from build123d import *

# Parameters (mm, degrees)
F1_DEPTH = 12.7
F2_R     = 9.525
F3_DEPTH = 34.29
F4_DEPTH = 25.4
F2_R_2   = 25.4
F5_DEPTH = 6.35


with BuildPart() as f1:
    # F0 (on Top) → F1 (new body)
    with BuildSketch(Plane.XY):
        Polygon((-48.986719159, 25.3412460777), (-50.7255351294, 24.7465363945), (-52.3601977854, 21.688304154), (-53.366815822, 18.3699267661), (-52.5578082129, 16.719871907), (-47.6057296253, 11.0468524364), (-43.80914346, 8.4974130761), (-42.2801519731, 7.9744654227), (-37.0147232049, 7.6171909331), (-33.782, 5.0679251692), (-33.782, -5.0679251692), (-37.0147232049, -7.6171909331), (-42.2801519731, -7.9744654227), (-43.80914346, -8.4974130761), (-47.6057296253, -11.0468524364), (-52.5578082129, -16.719871907), (-53.366815822, -18.3699267661), (-52.3601977854, -21.688304154), (-50.7255351294, -24.7465363945), (-48.986719159, -25.3412460777), (-41.4736370284, -25.8510271212), (-36.9863201834, -24.9691669416), (-35.5353802528, -24.2577827562), (-31.559527, -20.7871925925), (-27.4710453735, -20.303918365), (-20.303918365, -27.4710453735), (-20.7871925925, -31.559527), (-24.2577827562, -35.5353802528), (-24.9691669416, -36.9863201834), (-25.8510271212, -41.4736370284), (-25.3412460777, -48.986719159), (-24.7465363945, -50.7255351294), (-21.688304154, -52.3601977854), (-18.3699267661, -53.366815822), (-16.719871907, -52.5578082129), (-11.0468524364, -47.6057296253), (-8.4974130761, -43.80914346), (-7.9744654227, -42.2801519731), (-7.6171909331, -37.0147232049), (-5.0679251692, -33.782), (5.0679251692, -33.782), (7.6171909331, -37.0147232049), (7.9744654227, -42.2801519731), (8.4974130761, -43.80914346), (11.0468524364, -47.6057296253), (16.719871907, -52.5578082129), (18.3699267661, -53.366815822), (21.688304154, -52.3601977854), (24.7465363945, -50.7255351294), (25.3412460777, -48.986719159), (25.8510271212, -41.4736370284), (24.9691669416, -36.9863201834), (24.2577827562, -35.5353802528), (20.7871925925, -31.559527), (20.303918365, -27.4710453735), (27.4710453735, -20.303918365), (31.559527, -20.7871925925), (35.5353802528, -24.2577827562), (36.9863201834, -24.9691669416), (41.4736370284, -25.8510271212), (48.986719159, -25.3412460777), (50.7255351294, -24.7465363945), (52.3601977854, -21.688304154), (53.366815822, -18.3699267661), (52.5578082129, -16.719871907), (47.6057296253, -11.0468524364), (43.80914346, -8.4974130761), (42.2801519731, -7.9744654227), (37.0147232049, -7.6171909331), (33.782, -5.0679251692), (33.782, 5.0679251692), (37.0147232049, 7.6171909331), (42.2801519731, 7.9744654227), (43.80914346, 8.4974130761), (47.6057296253, 11.0468524364), (52.5578082129, 16.719871907), (53.366815822, 18.3699267661), (52.3601977854, 21.688304154), (50.7255351294, 24.7465363945), (48.986719159, 25.3412460777), (41.4736370284, 25.8510271212), (36.9863201834, 24.9691669416), (35.5353802528, 24.2577827562), (31.559527, 20.7871925925), (27.4710453735, 20.303918365), (20.303918365, 27.4710453735), (20.7871925925, 31.559527), (24.2577827562, 35.5353802528), (24.9691669416, 36.9863201834), (25.8510271212, 41.4736370284), (25.3412460777, 48.986719159), (24.7465363945, 50.7255351294), (21.688304154, 52.3601977854), (18.3699267661, 53.366815822), (16.719871907, 52.5578082129), (11.0468524364, 47.6057296253), (8.4974130761, 43.80914346), (7.9744654227, 42.2801519731), (7.6171909331, 37.0147232049), (5.0679251692, 33.782), (-5.0679251692, 33.782), (-7.6171909331, 37.0147232049), (-7.9744654227, 42.2801519731), (-8.4974130761, 43.80914346), (-11.0468524364, 47.6057296253), (-16.719871907, 52.5578082129), (-18.3699267661, 53.366815822), (-21.688304154, 52.3601977854), (-24.7465363945, 50.7255351294), (-25.3412460777, 48.986719159), (-25.8510271212, 41.4736370284), (-24.9691669416, 36.9863201834), (-24.2577827562, 35.5353802528), (-20.7871925925, 31.559527), (-20.303918365, 27.4710453735), (-27.4710453735, 20.303918365), (-31.559527, 20.7871925925), (-35.5353802528, 24.2577827562), (-36.9863201834, 24.9691669416), (-41.4736370284, 25.8510271212), align=None)
        Polygon((-6.457554456, 6.1279886028), (-5.0423575535, 7.3366771559), (-3.4067913067, 8.2247200336), (-1.622328418, 8.7533028893), (0.2330374214, 8.8993240645), (2.0782189459, 8.6564005578), (3.8325695574, 8.0351529003), (5.4194220185, 7.0627288788), (6.7694179402, 5.7816284228), (7.8235568446, 4.247847459), (8.5357689507, 2.5284119549), (8.8749315621, 0.6984712932), (8.8262133252, -1.1619911548), (8.3917463583, -2.9716744665), (7.5905194232, -4.6514766054), (6.457554456, -6.1279886028), (5.0423575535, -7.3366771559), (3.4067913067, -8.2247200336), (1.622328418, -8.7533028893), (-0.2330374214, -8.8993240645), (-2.0782189459, -8.6564005578), (-3.8325695574, -8.0351529003), (-5.4194220185, -7.0627288788), (-6.7694179402, -5.7816284228), (-7.8235568446, -4.247847459), (-8.5357689507, -2.5284119549), (-8.8749315621, -0.6984712932), (-8.8262133252, 1.1619911548), (-8.3917463583, 2.9716744665), (-7.5905194232, 4.6514766054), align=None, mode=Mode.SUBTRACT)
        Polygon((-3.4067913067, 8.2247200336), (-5.0423575535, 7.3366771559), (-6.457554456, 6.1279886028), (-7.5905194232, 4.6514766054), (-8.3917463583, 2.9716744665), (-8.8262133252, 1.1619911548), (-8.8749315621, -0.6984712932), (-8.5357689507, -2.5284119549), (-7.8235568446, -4.247847459), (-6.7694179402, -5.7816284228), (-5.4194220185, -7.0627288788), (-3.8325695574, -8.0351529003), (-2.0782189459, -8.6564005578), (-0.2330374214, -8.8993240645), (1.622328418, -8.7533028893), (3.4067913067, -8.2247200336), (5.0423575535, -7.3366771559), (6.457554456, -6.1279886028), (7.5905194232, -4.6514766054), (8.3917463583, -2.9716744665), (8.8262133252, -1.1619911548), (8.8749315621, 0.6984712932), (8.5357689507, 2.5284119549), (7.8235568446, 4.247847459), (6.7694179402, 5.7816284228), (5.4194220185, 7.0627288788), (3.8325695574, 8.0351529003), (2.0782189459, 8.6564005578), (0.2330374214, 8.8993240645), (-1.622328418, 8.7533028893), align=None)
    extrude(amount=F1_DEPTH)

    # F2 (on face) → F3 (join)
    with BuildSketch(Plane.XY.offset(12.7)):
        Circle(F2_R)
        with BuildLine():
            ThreePointArc((1.7960512242, 2.921), (2.9930503377, 1.6732276223), (3.429, 0))
            ThreePointArc((3.429, 0), (-1.6732276223, -2.9930503377), (-1.7960512242, 2.921))
            ThreePointArc((-1.7960512242, 2.921), (0, 3.429), (1.7960512242, 2.921))
        make_face(mode=Mode.SUBTRACT)
        with BuildLine():
            Line((-1.7960512242, 2.921), (1.7960512242, 2.921))
            ThreePointArc((1.7960512242, 2.921), (0, 3.429), (-1.7960512242, 2.921))
        make_face()
    extrude(amount=F3_DEPTH)

    # F4 (cut): a face of the model
    f4_faces = [f1.faces().sort_by_distance(p)[0] for p in [
        (0, -0.108182678, 12.7),
    ]]
    extrude(f4_faces, amount=-F4_DEPTH, mode=Mode.SUBTRACT)

    # F2 (on face) → F5 (cut)
    with BuildSketch(Plane.XY.offset(12.7)):
        Circle(F2_R_2)
        Circle(F2_R, mode=Mode.SUBTRACT)
    extrude(amount=-F5_DEPTH, mode=Mode.SUBTRACT)


solid = f1.part
Can you work these out from the model? Positions are in its coordinate system, mm. A direction names the side the tool comes from. Round coordinates to 2 decimals unless told otherwise and drop trailing zeros. Loops run counter-clockwise (first coordinate to the right, second up) from the corner with the lowest first, then second, coordinate; pieces in that order, holes last. Notation, with made-up numbers: (17.25, -35.75) - (46.25, -35.75) arc R28 ccw to (46.25, -3.75) - close; hole circle Ø4 at (-12.5, 13.5). An arc over 180 degrees is marked (long way). Answer in a Markdown table with one row per item. Add a question column.
Q1. Which directions (+Z, -Z, +X, -X, +Y, -Y) give clear straight access to the entire face, cutting with the end or side of a thin tool? Please do faces 1 (the flat face through (45.681, 9.754, 6.261)), 2 (the flat face through (29.487, -20.542, 6.261)), 3 (the flat face through (-35.376, -6.325, 6.261)).
Q2. I need wall thicknesses on L1, parallel to Y at x = 0, z = 8 (3 decimals); L2, parallel to Y at x = 0, z = 34 (3 decimals); L3, parallel to Z at x = 8.5, y = 32.5. Which ranges of each line are inside material? Lowest first, please.
Q3. We'd pull the mould along X, two halves only. Please class faces 4 (the flat face through (20.55, -29.54, 6.26)), 5 (the flat face through (-51.53, 23.24, 6.26)), 6 (the flat face through (0, 33.782, 6)): pulls with the +X half, pulls with the -X half, needs draft (parallel to the pull), parting line crosses it, or undercut.
Q4. I want a section at A-A on x = 0. List the corners of the cut face in (y, z) for me (3 decimals), and give its area (3 significant figures).
Q5. For pin 1 Ø1.1 at (x, z) = (0.5, 14.5) entering from -Y (3 decimals); pin 2 Ø12 at (y, z) = (7, 40) entering from -X; pin 3 Ø5 at (x, z) = (0.5, 8.5) entering from -Y, each with a flat end and sliding along its axis, tell me the tip position at first contact or that it passes through.
A:
| question | item | result |
|---|---|---|
| 1 | face 1 | +Z, -Z, +X |
| 1 | face 2 | +Z, -Z, -Y |
| 1 | face 3 | +Z, -Z, -X |
| 2 | L1 | -33.782 to -25.4, -9.525 to -3.429, 2.921 to 9.525, 25.4 to 33.782 |
| 2 | L2 | -9.525 to -3.429, 2.921 to 9.525 |
| 2 | L3 | 0 to 12.7 |
| 3 | face 4 | pulls with the +X half |
| 3 | face 5 | pulls with the -X half |
| 3 | face 6 | undercut |
| 4 | outline | (-33.782, 0) - (-3.429, 0) - (-3.429, 46.99) - (-9.525, 46.99) - (-9.525, 6.35) - (-25.4, 6.35) - (-25.4, 12.7) - (-33.782, 12.7) - close; (2.921, 0) - (33.782, 0) - (33.782, 12.7) - (25.4, 12.7) - (25.4, 6.35) - (9.525, 6.35) - (9.525, 46.99) - (2.921, 46.99) - close |
| 4 | area | 1,010 mm^2 |
| 5 | pin 1 | y = -9.525 |
| 5 | pin 2 | x = -9.47 |
| 5 | pin 3 | y = -33.78 |
